Check sheet for the modelled part. Datum: model origin and axes. Units: mm. Face numbers are marked on the shaded views. A direction names the side the tool comes from. Round coordinates to 2 decimals unless told otherwise and drop trailing zeros. Loops run counter-clockwise (first coordinate to the right, second up) from the corner with the lowest first, then second, coordinate; pieces in that order, holes last. Notation, with made-up numbers: (85, 45) - (133, 45) arc R14 cw to (133, 51) - close; hole circle Ø2 at (-6, 22.25). An arc over 180 degrees is marked (long way). Put each result on its own line as item: value. Start each with the question number.
Item 1: Section check C-C, the plane x = 10.5. Record the cut outline in (y, z).
Item 2: Material ranges on line 1 along X through (y, z) = (-6, 5.25); line 2 along Z through (x, y) = (15.5, 9.5); line 3 along X through (y, z) = (10, -2), recorded low to high.
Item 3: Section check A-A, the plane z = 15. Record the cut outline in (x, y).
Item 4: Tool access check on the marked faces 4 and 5. Record the directions out of +Z, -Z, +X, -X, +Y, -Y that give a thin tool (end or side, any length) a straight path to the whole face; none if there is none.
Item 5: Draft check along X on the marked faces 1, 2 and 3. Enter one of: pulls with the +X half, pulls with the -X half, needs draft (parallel to the pull), parting line crosses it, or undercut.
Item 6: Section check B-B, the plane z = 3.75. Record the cut outline in (x, y), and give its area (3 significant figures).
Item 7: Gauge pin test, flat ends, axial feed: pin 1 Ø1.5 at (x, y) = (-15.5, -10) entering from +Z; pin 2 Ø1.5 at (y, z) = (9.5, -2) entering from +X; pin 3 Ø0.9 at (y, z) = (-18.5, -1.5) entering from +X. Record the tip position at first contact, or that the pin passes through.
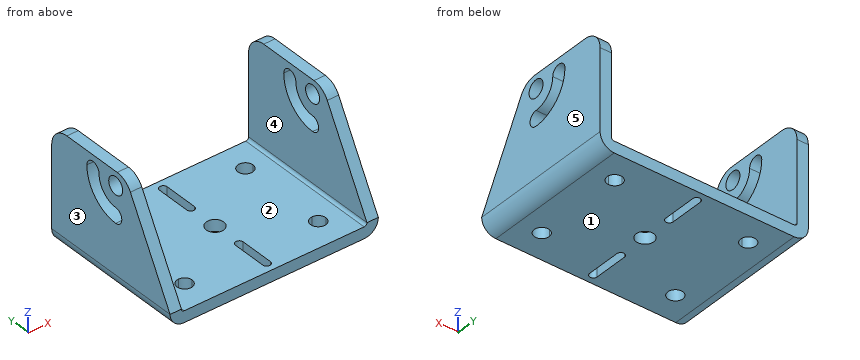
from build123d import *

# Parameters (mm, degrees)
ESBO_O1_W                        = 49
ESBO_O1_H                        = 39
FLANGE_BASE1_DEPTH               = 3
ESBO_O6_R                        = 2.3
CORTE_EXTRUS_O1_DEPTH            = 10
ARESTA_FLANGE1_STRIP_W           = 13.4732
ARESTA_FLANGE1_STRIP_H           = 3
ARESTA_FLANGE1_STRIP_CUT_DEPTH   = 39
ARESTA_FLANGE1_STRIP_2_W         = 13.4732
ARESTA_FLANGE1_STRIP_2_H         = 3
ARESTA_FLANGE1_STRIP_CUT_2_DEPTH = 39
ARESTA_FLANGE1_DEPTH             = 39
ARESTA_FLANGE1_BEND_DEPTH        = 39
ESBO_O13_R                       = 2.3
CORTE_EXTRUS_O2_DEPTH            = 70
FILETE1_R                        = 5


# Sheet-metal steps are written as plain solids
with BuildPart() as part:
    # Esboço1 → Flange-base1 (new body)
    with BuildSketch(Plane.XY):
        with Locations((2.493735783, -4.490936556)):
            Rectangle(ESBO_O1_W, ESBO_O1_H)
    extrude(amount=-FLANGE_BASE1_DEPTH)

    # Esboço6 → Corte-extrusão1 (cut)
    with BuildSketch(Plane.XY):
        with BuildLine():
            Line((-15.156264217, 5.509063444), (-15.156264217, 7.509063444))
            Line((-15.156264217, 7.509063444), (-13.156264217, 7.509063444))
            ThreePointArc((-13.156264217, 7.509063444), (-16.570477779, 8.923277006), (-15.156264217, 5.509063444))
        make_face()
        with BuildLine():
            Line((-13.156264217, 7.509063444), (-15.156264217, 7.509063444))
            Line((-15.156264217, 7.509063444), (-15.156264217, 5.509063444))
            ThreePointArc((-15.156264217, 5.509063444), (-13.742050654, 6.094849882), (-13.156264217, 7.509063444))
        make_face()
        with BuildLine():
            ThreePointArc((-13.156264217, -16.490936556), (-13.742050654, -15.076722994), (-15.156264217, -14.490936556))
            Line((-15.156264217, -14.490936556), (-15.156264217, -16.490936556))
            Line((-15.156264217, -16.490936556), (-13.156264217, -16.490936556))
        make_face()
        with BuildLine():
            Line((-15.156264217, -16.490936556), (-15.156264217, -14.490936556))
            ThreePointArc((-15.156264217, -14.490936556), (-16.570477779, -17.905150118), (-13.156264217, -16.490936556))
            Line((-13.156264217, -16.490936556), (-15.156264217, -16.490936556))
        make_face()
        with Locations((2.493735783, -4.490936556)):
            Circle(ESBO_O6_R)
        with BuildLine():
            Line((3.493735783, 7.509063444), (1.493735783, 7.509063444))
            Line((1.493735783, 7.509063444), (1.493735783, 3.523823043))
            ThreePointArc((1.493735783, 3.523823043), (2.493735783, 2.523823043), (3.493735783, 3.523823043))
            Line((3.493735783, 3.523823043), (3.493735783, 7.509063444))
        make_face()
        with BuildLine():
            Line((1.493735783, 12.523823043), (1.493735783, 7.509063444))
            Line((1.493735783, 7.509063444), (3.493735783, 7.509063444))
            Line((3.493735783, 7.509063444), (3.493735783, 12.523823043))
            ThreePointArc((3.493735783, 12.523823043), (2.493735783, 13.523823043), (1.493735783, 12.523823043))
        make_face()
        with BuildLine():
            Line((1.493735783, -12.505696155), (1.493735783, -16.490936556))
            Line((1.493735783, -16.490936556), (3.493735783, -16.490936556))
            Line((3.493735783, -16.490936556), (3.493735783, -12.505696155))
            ThreePointArc((3.493735783, -12.505696155), (2.493735783, -11.505696155), (1.493735783, -12.505696155))
        make_face()
        with BuildLine():
            Line((3.493735783, -16.490936556), (1.493735783, -16.490936556))
            Line((1.493735783, -16.490936556), (1.493735783, -21.505696155))
            ThreePointArc((1.493735783, -21.505696155), (2.493735783, -22.505696155), (3.493735783, -21.505696155))
            Line((3.493735783, -21.505696155), (3.493735783, -16.490936556))
        make_face()
        with BuildLine():
            ThreePointArc((22.143735783, -16.490936556), (21.557949346, -15.076722994), (20.143735783, -14.490936556))
            Line((20.143735783, -14.490936556), (20.143735783, -16.490936556))
            Line((20.143735783, -16.490936556), (18.143735783, -16.490936556))
            ThreePointArc((18.143735783, -16.490936556), (20.143735783, -18.490936556), (22.143735783, -16.490936556))
        make_face()
        with BuildLine():
            Line((20.143735783, -16.490936556), (20.143735783, -14.490936556))
            ThreePointArc((20.143735783, -14.490936556), (18.729522221, -15.076722994), (18.143735783, -16.490936556))
            Line((18.143735783, -16.490936556), (20.143735783, -16.490936556))
        make_face()
        with BuildLine():
            ThreePointArc((22.143735783, 7.509063444), (20.143735783, 9.509063444), (18.143735783, 7.509063444))
            Line((18.143735783, 7.509063444), (20.143735783, 7.509063444))
            Line((20.143735783, 7.509063444), (20.143735783, 5.509063444))
            ThreePointArc((20.143735783, 5.509063444), (21.557949346, 6.094849882), (22.143735783, 7.509063444))
        make_face()
        with BuildLine():
            Line((20.143735783, 7.509063444), (18.143735783, 7.509063444))
            ThreePointArc((18.143735783, 7.509063444), (18.729522221, 6.094849882), (20.143735783, 5.509063444))
            Line((20.143735783, 5.509063444), (20.143735783, 7.509063444))
        make_face()
    extrude(amount=-CORTE_EXTRUS_O1_DEPTH, mode=Mode.SUBTRACT)

    # Aresta-Flange1 strip (across the edge) → Aresta-Flange1 strip cut (cut)
    with BuildSketch(Plane(origin=(26.993735783, -23.990936556, 0), x_dir=(-1, 0, 0), z_dir=(0, 1, 0))):
        with Locations((-6, -1.5)):
            Rectangle(ARESTA_FLANGE1_STRIP_W, ARESTA_FLANGE1_STRIP_H)
    extrude(amount=ARESTA_FLANGE1_STRIP_CUT_DEPTH, mode=Mode.SUBTRACT)

    # Aresta-Flange1 strip 2 (across the edge) → Aresta-Flange1 strip cut 2 (cut)
    with BuildSketch(Plane(origin=(-22.006264217, 15.009063444, 0), x_dir=(1, 0, 0), z_dir=(0, -1, 0))):
        with Locations((-6, -1.5)):
            Rectangle(ARESTA_FLANGE1_STRIP_2_W, ARESTA_FLANGE1_STRIP_2_H)
    extrude(amount=ARESTA_FLANGE1_STRIP_CUT_2_DEPTH, mode=Mode.SUBTRACT)

    # Aresta-Flange1 section (across the edge) → Aresta-Flange1 (add)
    with BuildSketch(Plane(origin=(26.993735783, -23.990936556, 0), x_dir=(-1, 0, 0), z_dir=(0, 1, 0))):
        with BuildLine():
            Line((-3, 0.7366), (-3, 27))
            Line((-3, 27), (0, 27))
            Line((0, 27), (0, 0.7366))
            ThreePointArc((0, 0.7366), (0.215745145, 0.215745145), (0.7366, 0))
            Line((0.7366, 0), (0.7366, -3))
            ThreePointArc((0.7366, -3), (-1.905575199, -1.905575199), (-3, 0.7366))
        make_face()
    extrude(amount=ARESTA_FLANGE1_DEPTH)

    # Aresta-Flange1 section 2 (across the edge) → Aresta-Flange1 bend (add)
    with BuildSketch(Plane(origin=(-22.006264217, 15.009063444, 0), x_dir=(1, 0, 0), z_dir=(0, -1, 0))):
        with BuildLine():
            Line((-3, 0.7366), (-3, 27))
            Line((-3, 27), (0, 27))
            Line((0, 27), (0, 0.7366))
            ThreePointArc((0, 0.7366), (0.215745145, 0.215745145), (0.7366, 0))
            Line((0.7366, 0), (0.7366, -3))
            ThreePointArc((0.7366, -3), (-1.905575199, -1.905575199), (-3, 0.7366))
        make_face()
    extrude(amount=ARESTA_FLANGE1_BEND_DEPTH)

    # Esboço13 → Corte-extrusão2 (cut)
    with BuildSketch(Plane.ZY.offset(25.006264217)):
        with Locations((23.343855314, -6.08027591)):
            Circle(ESBO_O13_R)
        Polygon((0.7366, -23.990936556), (27, -23.990936556), (27, -9.490936556), align=None)
        with BuildLine():
            ThreePointArc((23.343855314, 3.41972409), (16.626340893, 0.637238511), (13.843855314, -6.08027591))
            ThreePointArc((13.843855314, -6.08027591), (15.843855314, -8.08027591), (17.843855314, -6.08027591))
            ThreePointArc((17.843855314, -6.08027591), (19.454768018, -2.191188614), (23.343855314, -0.58027591))
            ThreePointArc((23.343855314, -0.58027591), (25.343855314, 1.41972409), (23.343855314, 3.41972409))
        make_face()
    extrude(amount=-CORTE_EXTRUS_O2_DEPTH, mode=Mode.SUBTRACT)

    # Filete1
    filete1_edges = [part.edges().sort_by_distance(p)[0] for p in [
        (28.493735783, 15.009063444, 27),
        (-23.506264217, 15.009063444, 27),
        (-23.506264217, -9.490936556, 27),
        (28.493735783, -9.490936556, 27),
    ]]
    fillet(filete1_edges, radius=FILETE1_R)


solid = part.part
Check result:
1. outline: (-23.99, -3) - (15.01, -3) - (15.01, 0) - (-23.99, 0) - close
2. line 1: -25.01 to -22.01, 26.99 to 29.99
2. line 2: -3 to 0
2. line 3: -23.81 to 1.49, 3.49 to 28.8
3. outline: (-25.01, -16.12) - (-22.01, -16.12) - (-22.01, -7.89) - (-25.01, -7.89) - close; (-25.01, -1.54) - (-22.01, -1.54) - (-22.01, 15.01) - (-25.01, 15.01) - close; (26.99, -16.12) - (29.99, -16.12) - (29.99, -7.89) - (26.99, -7.89) - close; (26.99, -1.54) - (29.99, -1.54) - (29.99, 15.01) - (26.99, 15.01) - close
4. face 4: +Z, +Y, -Y
4. face 5: +Z, -Z, +X, +Y, -Y
5. face 1: needs draft
5. face 2: undercut
5. face 3: pulls with the -X half
6. outline: (-25.01, -22.33) - (-22.01, -22.33) - (-22.01, 15.01) - (-25.01, 15.01) - close; (26.99, -22.33) - (29.99, -22.33) - (29.99, 15.01) - (26.99, 15.01) - close
6. area: 224 mm²
7. pin 1: z = 0
7. pin 2: x = 29.42
7. pin 3: x = 29.54
